Could you check a few things on this drawing? It's one solid part, dimensions in mm from its lowest x, y, z. A direction names the side the tool comes from. Give positions to 0.01 mm unless a question says otherwise; leave off trailing zeros. Loops run counter-clockwise (first coordinate to the right, second up) from the corner with the lowest first, then second, coordinate; pieces in that order, holes last. Notation, with made-up numbers: (6.25, 8) - (43.25, 8) arc R15 ccw to (43.25, 35) - close; hole circle Ø4 at (42, 20). An arc over 180 degrees is marked (long way). Write item = value, one per line.
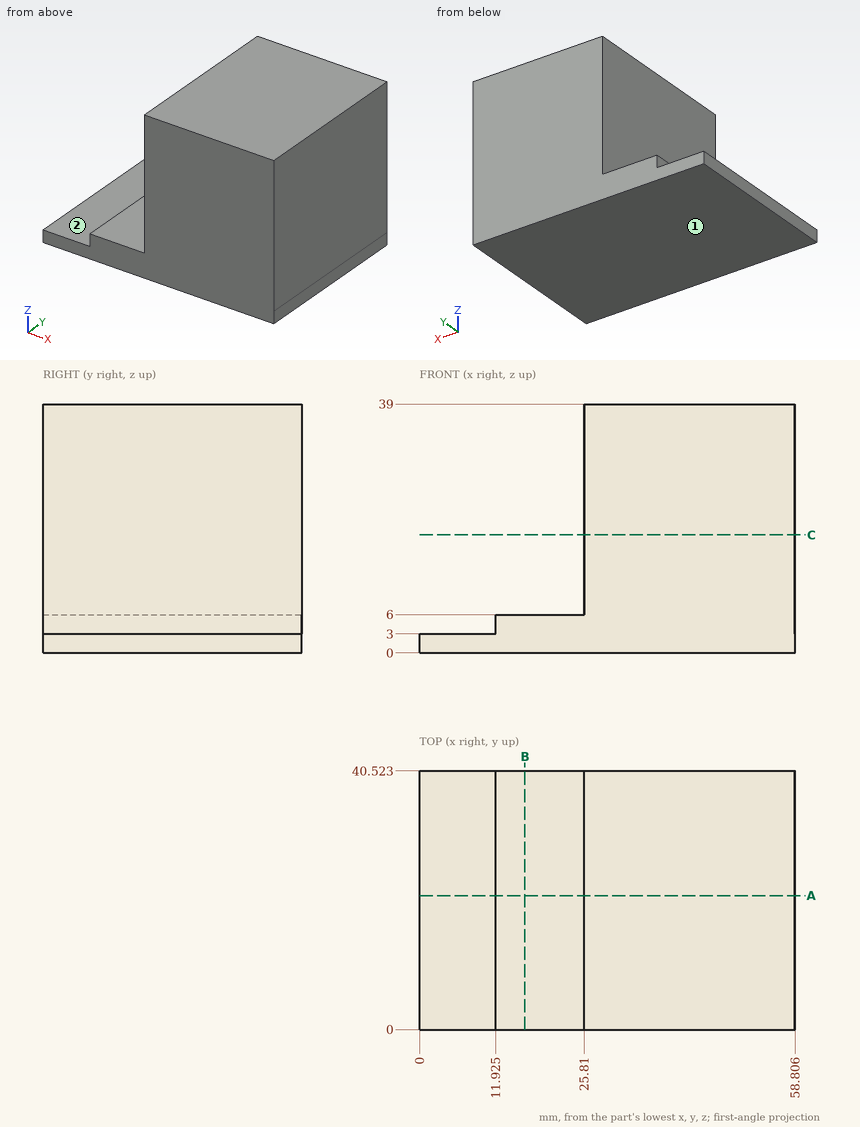
Q1. Imagine slicing it at B-B, the plane x = 16.5. Write out the boundary of the cut face in (y, z).
Output:
outline = (0, 0) - (40.52, 0) - (40.52, 6) - (0, 6) - close
Q2. Imagine slicing it at A-A, the plane y = 21. Write out the boundary of the cut face in (x, z) (1 decimal), then the cut area to 3 significant figures.
Output:
outline = (0, 0) - (58.8, 0) - (58.8, 39) - (25.8, 39) - (25.8, 6) - (11.9, 6) - (11.9, 3) - (0, 3) - close
area = 1,410 mm2
Q3. I need wall thicknesses on L1, parallel to X at y = 5.5, z = 9.5; L2, parallel to Z at x = 3.5, y = 33; L3, parallel to Z at x = 25, y = 2.5. Which ranges of each line are inside material? Lowest first, please.
Output:
L1 = 25.81 to 58.81
L2 = 0 to 3
L3 = 0 to 6
Q4. For pin 1 (1.5 mm diameter, centred on y = 23, z = 4.5, fed in from -X) (1 decimal); pin 2 (10 mm diameter, centred on y = 27, z = 18, fed in from -X); pin 3 (6 mm diameter, centred on x = 9, y = 20.5, fed in from +Z), each with a flat end and sliding along its axis, tell me the tip position at first contact or that it passes through.
Output:
pin_1 = 11.9
pin_2 = 25.81
pin_3 = 6
Q5. Which directions (+Z, -Z, +X, -X, +Y, -Y) give clear straight access to the entire face, cutting with the end or side of a thin tool? Please do the marked faces 1 and 2.
Output:
face_1 = -Z, +X, -X, +Y, -Y
face_2 = +Z, -X, +Y, -Y
Q6. Imagine slicing it at C-C, the plane z = 18.5. Write out the boundary of the cut face in (x, y).
Output:
outline = (25.81, 0) - (58.81, 0) - (58.81, 40.52) - (25.81, 40.52) - close
